from build123d import *

# Parameters (mm, degrees)
SKETCH_1_R           = 1.25
EXTRUDE_1_DEPTH      = 3
SKETCH_2_R           = 1.5
CUT_EXTRUDE_1_DEPTH  = 3
CUT_EXTRUDE_2_DEPTH  = 3
CUT_EXTRUDE_3_DEPTH  = 3
CUT_EXTRUDE_4_DEPTH  = 10
SKETCH_6_R           = 1.5
CUT_EXTRUDE_5_DEPTH  = 10
SKETCH_7_R           = 1.5
CUT_EXTRUDE_8_DEPTH  = 10
SKETCH_8_R           = 1.5
CUT_EXTRUDE_9_DEPTH  = 10
SKETCH_9_R           = 15
CUT_EXTRUDE_10_DEPTH = 10
SKETCH_10_R          = 1.5
CUT_EXTRUDE_11_DEPTH = 10
CUT_EXTRUDE_12_DEPTH = 10


with BuildPart() as part:
    # 草图1 → 凸台-拉伸1 (new body)
    # profile 1 of 4: a face of its own
    with BuildSketch(Plane(origin=(0, 0, 0), x_dir=(1, 0, 0), z_dir=(0, 1, 0))):
        with BuildLine():
            ThreePointArc((75, -15), (32.573593129, -32.573593129), (15, -75))
            Line((15, -75), (0, -75))
            Line((0, -75), (0, 0))
            Line((0, 0), (75, 0))
            Line((75, 0), (75, -15))
        make_face()
        with Locations(Location((11, -70, 0), (0, 0, 270))):
            Circle(SKETCH_1_R, mode=Mode.SUBTRACT)
        with Locations(Location((70, -11, 0), (0, 0, 270))):
            Circle(SKETCH_1_R, mode=Mode.SUBTRACT)
    # profile 2 of 4: a face of its own
    with BuildSketch(Plane(origin=(0, 0, 0), x_dir=(1, 0, 0), z_dir=(0, 1, 0))):
        with BuildLine():
            ThreePointArc((-15, -75), (-32.573593129, -32.573593129), (-75, -15))
            Line((-75, -15), (-75, 0))
            Line((-75, 0), (0, 0))
            Line((0, 0), (0, -75))
            Line((0, -75), (-15, -75))
        make_face()
        with Locations(Location((-70, -11, 0), (0, 0, 270))):
            Circle(SKETCH_1_R, mode=Mode.SUBTRACT)
        with Locations(Location((-11, -70, 0), (0, 0, 270))):
            Circle(SKETCH_1_R, mode=Mode.SUBTRACT)
    # profile 3 of 4: a face of its own
    with BuildSketch(Plane(origin=(0, 0, 0), x_dir=(1, 0, 0), z_dir=(0, 1, 0))):
        with BuildLine():
            ThreePointArc((-75, 15), (-32.573593129, 32.573593129), (-15, 75))
            Line((-15, 75), (0, 75))
            Line((0, 75), (0, 0))
            Line((0, 0), (-75, 0))
            Line((-75, 0), (-75, 15))
        make_face()
        with Locations(Location((-11, 70, 0), (0, 0, 270))):
            Circle(SKETCH_1_R, mode=Mode.SUBTRACT)
        with Locations(Location((-70, 11, 0), (0, 0, 270))):
            Circle(SKETCH_1_R, mode=Mode.SUBTRACT)
    # profile 4 of 4: a face of its own
    with BuildSketch(Plane(origin=(0, 0, 0), x_dir=(1, 0, 0), z_dir=(0, 1, 0))):
        with BuildLine():
            ThreePointArc((15, 75), (32.573593129, 32.573593129), (75, 15))
            Line((75, 15), (75, 0))
            Line((75, 0), (0, 0))
            Line((0, 0), (0, 75))
            Line((0, 75), (15, 75))
        make_face()
        with Locations(Location((70, 11, 0), (0, 0, 270))):
            Circle(SKETCH_1_R, mode=Mode.SUBTRACT)
        with Locations(Location((11, 70, 0), (0, 0, 270))):
            Circle(SKETCH_1_R, mode=Mode.SUBTRACT)
    extrude(amount=EXTRUDE_1_DEPTH)

    # 草图2 → 切除-拉伸1 (cut)
    with BuildSketch(Plane.XZ):
        with Locations(Location((0.353553391, -31.466251763, 0), (0, 0, 270))):
            Circle(SKETCH_2_R)
        with Locations(Location((31.466251763, -0.353553391, 0), (0, 0, 270))):
            Circle(SKETCH_2_R)
        with Locations(Location((-0.353553391, 31.466251763, 0), (0, 0, 90))):
            Circle(SKETCH_2_R)
        with Locations(Location((-31.466251763, 0.353553391, 0), (0, 0, 90))):
            Circle(SKETCH_2_R)
    extrude(amount=-CUT_EXTRUDE_1_DEPTH, mode=Mode.SUBTRACT)

    # 草图3 → 切除-拉伸2 (cut)
    with BuildSketch(Plane(origin=(0, 3, 0), x_dir=(1, 0, 0), z_dir=(0, 1, 0))):
        Polygon((-15.556349186, 15.556349186), (-12.02081528, 19.091883092), (-22.627416998, 22.627416998), align=None)
        Polygon((-19.091883092, 12.02081528), (-15.556349186, 15.556349186), (-22.627416998, 22.627416998), align=None)
    extrude(amount=-CUT_EXTRUDE_2_DEPTH, mode=Mode.SUBTRACT)

    # 草图4 → 切除-拉伸3 (cut)
    with BuildSketch(Plane(origin=(0, 3, 0), x_dir=(1, 0, 0), z_dir=(0, 1, 0))):
        with BuildLine():
            ThreePointArc((33.944668714, -19.80253309), (34.043922781, -8.582763971), (22.827665534, -8.285032838))
            Line((22.827665534, -8.285032838), (15.556349186, -15.556349186))
            Line((15.556349186, -15.556349186), (8.285032838, -22.827665534))
            ThreePointArc((8.285032838, -22.827665534), (8.582763971, -34.043922781), (19.80253309, -33.944668714))
            Line((19.80253309, -33.944668714), (33.944668714, -19.80253309))
        make_face()
    extrude(amount=-CUT_EXTRUDE_3_DEPTH, mode=Mode.SUBTRACT)

    # 草图5 → 切除-拉伸4 (cut)
    with BuildSketch(Plane(origin=(0, 3, 0), x_dir=(1, 0, 0), z_dir=(0, 1, 0))):
        Polygon((-22.627416998, 8.485281374), (-22.627416998, 22.627416998), (-19.091883092, 12.02081528), align=None)
        Polygon((-12.02081528, 19.091883092), (-22.627416998, 22.627416998), (-8.485281374, 22.627416998), align=None)
    extrude(amount=-CUT_EXTRUDE_4_DEPTH, mode=Mode.SUBTRACT)

    # 草图6 → 切除-拉伸5 (cut)
    with BuildSketch(Plane(origin=(0, 3, 0), x_dir=(1, 0, 0), z_dir=(0, 1, 0))):
        with Locations(Location((-35.355339059, -21.213203436, 0), (0, 0, 270))):
            Circle(SKETCH_6_R)
        with Locations(Location((-21.213203436, -35.355339059, 0), (0, 0, 270))):
            Circle(SKETCH_6_R)
        with Locations(Location((35.355339059, 21.213203436, 0), (0, 0, 270))):
            Circle(SKETCH_6_R)
        with Locations(Location((21.213203436, 35.355339059, 0), (0, 0, 270))):
            Circle(SKETCH_6_R)
    extrude(amount=-CUT_EXTRUDE_5_DEPTH, mode=Mode.SUBTRACT)

    # 草图7 → 切除-拉伸8 (cut)
    with BuildSketch(Plane(origin=(0, 3, 0), x_dir=(1, 0, 0), z_dir=(0, 1, 0))):
        with Locations(Location((-29.69848481, 29.69848481, 0), (0, 0, 270))):
            Circle(SKETCH_7_R)
        with Locations(Location((29.69848481, 29.69848481, 0), (0, 0, 270))):
            Circle(SKETCH_7_R)
        with Locations(Location((29.69848481, -29.69848481, 0), (0, 0, 270))):
            Circle(SKETCH_7_R)
        with Locations(Location((-29.69848481, -29.69848481, 0), (0, 0, 270))):
            Circle(SKETCH_7_R)
    extrude(amount=-CUT_EXTRUDE_8_DEPTH, mode=Mode.SUBTRACT)

    # 草图8 → 切除-拉伸9 (cut)
    with BuildSketch(Plane(origin=(0, 3, 0), x_dir=(1, 0, 0), z_dir=(0, 1, 0))):
        with Locations(Location((-11, 55, 0), (0, 0, 270))):
            Circle(SKETCH_8_R)
        with Locations(Location((11, 55, 0), (0, 0, 270))):
            Circle(SKETCH_8_R)
        with Locations(Location((55, 11, 0), (0, 0, 270))):
            Circle(SKETCH_8_R)
        with Locations(Location((55, -11, 0), (0, 0, 270))):
            Circle(SKETCH_8_R)
        with Locations(Location((11, -55, 0), (0, 0, 270))):
            Circle(SKETCH_8_R)
        with Locations(Location((-11, -55, 0), (0, 0, 270))):
            Circle(SKETCH_8_R)
        with Locations(Location((-55, -11, 0), (0, 0, 270))):
            Circle(SKETCH_8_R)
        with Locations(Location((-55, 11, 0), (0, 0, 270))):
            Circle(SKETCH_8_R)
    extrude(amount=-CUT_EXTRUDE_9_DEPTH, mode=Mode.SUBTRACT)

    # 草图9 → 切除-拉伸10 (cut)
    with BuildSketch(Plane(origin=(0, 3, 0), x_dir=(1, 0, 0), z_dir=(0, 1, 0))):
        with Locations(Location((0, 0, 0), (0, 0, 270))):
            Circle(SKETCH_9_R)
    extrude(amount=-CUT_EXTRUDE_10_DEPTH, mode=Mode.SUBTRACT)

    # 草图10 → 切除-拉伸11 (cut)
    with BuildSketch(Plane(origin=(0, 3, 0), x_dir=(1, 0, 0), z_dir=(0, 1, 0))):
        with Locations(Location((11, 70, 0), (0, 0, 270))):
            Circle(SKETCH_10_R)
        with Locations(Location((-11, 70, 0), (0, 0, 270))):
            Circle(SKETCH_10_R)
        with Locations(Location((70, 11, 0), (0, 0, 270))):
            Circle(SKETCH_10_R)
        with Locations(Location((70, -11, 0), (0, 0, 270))):
            Circle(SKETCH_10_R)
        with Locations(Location((11, -70, 0), (0, 0, 270))):
            Circle(SKETCH_10_R)
        with Locations(Location((-11, -70, 0), (0, 0, 270))):
            Circle(SKETCH_10_R)
        with Locations(Location((-70, -11, 0), (0, 0, 270))):
            Circle(SKETCH_10_R)
        with Locations(Location((-70, 11, 0), (0, 0, 270))):
            Circle(SKETCH_10_R)
    extrude(amount=-CUT_EXTRUDE_11_DEPTH, mode=Mode.SUBTRACT)

    # 草图11 → 切除-拉伸12 (cut)
    with BuildSketch(Plane(origin=(0, 3, 0), x_dir=(1, 0, 0), z_dir=(0, 1, 0))):
        with BuildLine():
            Line((3, 70), (3, 55))
            ThreePointArc((3, 55), (0, 52), (-3, 55))
            Line((-3, 55), (-3, 70))
            ThreePointArc((-3, 70), (0, 73), (3, 70))
        make_face()
        with BuildLine():
            Line((70, -3), (55, -3))
            ThreePointArc((55, -3), (52, 0), (55, 3))
            Line((55, 3), (70, 3))
            ThreePointArc((70, 3), (73, 0), (70, -3))
        make_face()
        with BuildLine():
            Line((-3, -70), (-3, -55))
            ThreePointArc((-3, -55), (0, -52), (3, -55))
            Line((3, -55), (3, -70))
            ThreePointArc((3, -70), (0, -73), (-3, -70))
        make_face()
        with BuildLine():
            Line((-70, 3), (-55, 3))
            ThreePointArc((-55, 3), (-52, 0), (-55, -3))
            Line((-55, -3), (-70, -3))
            ThreePointArc((-70, -3), (-73, 0), (-70, 3))
        make_face()
    extrude(amount=-CUT_EXTRUDE_12_DEPTH, mode=Mode.SUBTRACT)


solid = part.part
Model file for the job. Use its own axes, mm. A direction names the side the tool comes from. Round coordinates to 2 decimals unless told otherwise and drop trailing zeros. Order: outer loops, then holes, each group sorted by start corner. A loop starts at its lowest first (then second) coordinate and runs counter-clockwise, first axis right, second up.
(1) Pin check, flat tips, straight feed: pin 1 (4 mm diameter, centred on x = 70, z = 11, fed in from -Y); pin 2 (2.5 mm diameter, centred on x = 11, z = 55, fed in from -Y). Stop position of each tip, or through.
(2) Pull direction X, two halves, no side cores. Call faces 1 (the face through (-16, 0, -1)), 2 (the face through (26.775, 1.521, 26.973)), 3 (the face through (-33.04, 1.48, -32.11)): released by +X, released by -X, zero draft, split by the parting line, or undercut.
(3) 3-axis set-ups, long thin cutter, end or side, ignore diameter. For faces 4 (the face through (32.11, 1.48, -33.04)), 5 (the face through (15.66, 1.52, 15.45)): which of +Z, -Z, +X, -X, +Y, -Y reach the whole face in a straight line?
(4) Drill centre lines: line 1 (X direction, y = 0.95, z = 55); line 2 (Z direction, x = -9, y = 1.85); line 3 (Z direction, x = 34.5, y = 0.3). Where is each one in solid material? Low to high.
(5) Band-saw the part on C-C (y = 2.3). Give the number of separate pieces and of enclosed holes in the cut face, then the cut area to 3 significant figures.
(6) Band-saw the part on B-B (x = 43.5). List the corners of the cut face in (y, z), then the cut area to 3 significant figures.
(7) Band-saw the part on A-A (z = 17). List the corners of the cut face in (x, y), then the cut area to 3 significant figures.
Verdict:
1. pin 1: stops at y = 0
1. pin 2: passes through
2. face 1: zero draft
2. face 2: undercut
2. face 3: released by -X
3. face 4: -Z, +X, +Y, -Y
3. face 5: +Y, -Y
4. line 1: x = -18.43 to -12.5, -9.5 to -3, 3 to 9.5, 12.5 to 18.43
4. line 2: z = -75 to -22.63, -22.11 to -12, 12 to 75
4. line 3: z = -30.73 to -22.45, -19.98 to 9.1, 19.19 to 30.73
5. separate pieces: 1
5. enclosed holes: 35
5. area: 9,190 mm2
6. outline: (0, -23.93) - (3, -23.93) - (3, 23.93) - (0, 23.93) - close
6. area: 144 mm2
7. outline: (-59.64, 0) - (14.11, 0) - (14.11, 3) - (-59.64, 3) - close; (35.76, 0) - (59.64, 0) - (59.64, 3) - (35.76, 3) - close
7. area: 293 mm2
